from build123d import *

# Parameters (mm, degrees)
EXTRUDE_1_DEPTH        = 4
SKETCH_2_W             = 36
SKETCH_2_H             = 8
CUT_EXTRUDE_1_DEPTH    = 1
SKETCH_3_R             = 1.9
CUT_EXTRUDE_2_DEPTH    = 3
PATTERN_LINEAR_1_COUNT = 5
PATTERN_LINEAR_1_PITCH = 8


with BuildPart() as part:
    # 草图1 → 凸台-拉伸1 (new body)
    with BuildSketch(Plane.XY):
        with BuildLine():
            Line((-12, 6), (12, 6))
            ThreePointArc((12, 6), (18, 0), (12, -6))
            Line((12, -6), (-12, -6))
            ThreePointArc((-12, -6), (-18, 0), (-12, 6))
        make_face()
    extrude(amount=EXTRUDE_1_DEPTH)

    # 草图2 → 切除-拉伸1 (cut)
    with BuildSketch(Plane.XY.offset(4)):
        Rectangle(SKETCH_2_W, SKETCH_2_H)
    extrude(amount=-CUT_EXTRUDE_1_DEPTH, mode=Mode.SUBTRACT)

    # 草图3 → 切除-拉伸2 (cut)
    with BuildSketch(Plane.XY.offset(3)):
        with Locations((-12, 0)):
            Circle(SKETCH_3_R)
    cut_extrude_2 = extrude(amount=-CUT_EXTRUDE_2_DEPTH, mode=Mode.SUBTRACT)

    # 阵列(线性)1: 切除-拉伸2 ×5
    with Locations(*[(i * PATTERN_LINEAR_1_PITCH, 0, 0) for i in range(1, PATTERN_LINEAR_1_COUNT)]):
        add(cut_extrude_2, mode=Mode.SUBTRACT)


solid = part.part
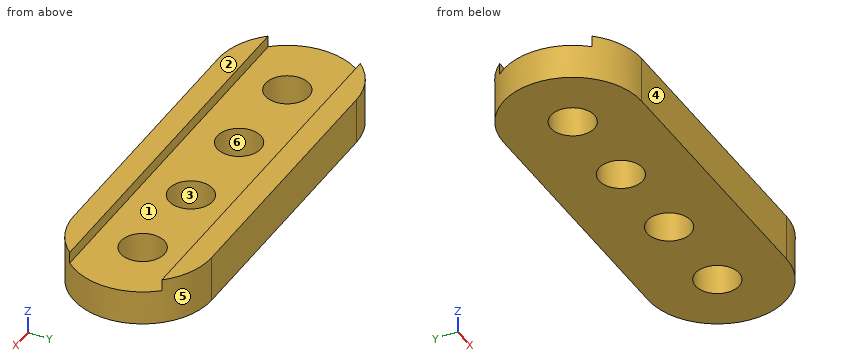
Geometry: final body of the model. Coordinates: model frame, mm. Face numbers are marked on the shaded views. A direction names the side the tool comes from. Coordinates: 2 decimals unless noted, no trailing zeros. Loops run counter-clockwise (first coordinate to the right, second up) from the corner with the lowest first, then second, coordinate; pieces in that order, holes last. Notation, with made-up numbers: (45.25, 68) - (104.25, 68) arc R12 cw to (104.25, 73) - close; hole circle Ø5 at (42, 30.25). An arc over 180 degrees is marked (long way). One line per question, with ' | ' between items. Start each with the question number.
(1) Reachability of the marked faces 1 and 2 from +Z, -Z, +X, -X, +Y, -Y: full face, straight path, thin tool, end or side. Return the list, or none.
(2) Cut plane B-B on y = 0. Output: boundary loops of the cut face in (x, z).
(3) Ray query, L1, parallel to Y at x = 4, z = 1.45; L2, parallel to Y at x = -5.5, z = 3.6; L3, parallel to X at y = -1.25, z = 1.85. Return the intervals inside material, ascending. Write a range as from..to.
(4) Cut plane C-C on z = 2.05. Output: boundary loops of the cut face in (x, y).
(5) Draft query along X for the marked faces 3, 4, 5 and 6. Return one class per face: +X half, -X half, draft (parallel to the pull), parting line (faces both ways), or undercut.
(6) First-contact query: pin 1 (2.5 mm diameter, centred on x = -3, y = 1.5, fed in from +Z); pin 2 (1.5 mm diameter, centred on y = -1, z = 2.5, fed in from -X). Flat tips, straight axial feed; report the tip coordinate or a pass-through.
(7) Cut plane A-A on x = 4. Output: boundary loops of the cut face in (y, z), and give its area (3 significant figures).
(8) Cut plane D-D on x = 8.5. Output: boundary loops of the cut face in (y, z), and give its area (3 significant figures).
Here are the results:
1) face 1: +Z, +X, -X | face 2: +Z, +X, -X, +Y, -Y
2) outline: (-18, 0) - (-13.9, 0) - (-13.9, 3) - (-18, 3) - close; (-10.1, 0) - (-5.9, 0) - (-5.9, 3) - (-10.1, 3) - close; (-2.1, 0) - (2.1, 0) - (2.1, 3) - (-2.1, 3) - close; (5.9, 0) - (10.1, 0) - (10.1, 3) - (5.9, 3) - close; (13.9, 0) - (18, 0) - (18, 3) - (13.9, 3) - close
3) L1: -6..-1.9, 1.9..6 | L2: -6..-4, 4..6 | L3: -17.87..-13.43, -10.57..-5.43, -2.57..2.57, 5.43..10.57, 13.43..17.87
4) outline: (-12, -6) - (12, -6) arc R6 ccw to (12, 6) - (-12, 6) arc R6 ccw to start; hole circle Ø3.8 at (-12, 0); hole circle Ø3.8 at (-4, 0); hole circle Ø3.8 at (4, 0); hole circle Ø3.8 at (12, 0)
5) face 3: undercut | face 4: draft | face 5: +X half | face 6: undercut
6) pin 1: z = 3 | pin 2: x = -17.99
7) outline: (-6, 0) - (-1.9, 0) - (-1.9, 3) - (-4, 3) - (-4, 4) - (-6, 4) - close; (1.9, 0) - (6, 0) - (6, 4) - (4, 4) - (4, 3) - (1.9, 3) - close | area: 28.6 mm²
8) outline: (-6, 0) - (6, 0) - (6, 4) - (4, 4) - (4, 3) - (-4, 3) - (-4, 4) - (-6, 4) - close | area: 40.0 mm²
